from build123d import *

# Parameters (mm, degrees)
F0_R     = 3.663821
F0_R_2   = 3.4798
F1_DEPTH = 3.175


with BuildPart() as f1:
    # F0 (on Top) → F1 (new body)
    with BuildSketch(Plane.XY):
        with BuildLine():
            ThreePointArc((-89.269999, -19.05), (-87.410127, -23.540128), (-82.919999, -25.4))
            Line((-82.919999, -25.4), (56.780001, -25.4))
            ThreePointArc((56.780001, -25.4), (61.270129, -23.540128), (63.130001, -19.05))
            Line((63.130001, -19.05), (63.130001, -6.35))
            ThreePointArc((63.130001, -6.35), (61.270129, -1.859872), (56.780001, 0))
            Line((56.780001, 0), (-9.894999, 0))
            ThreePointArc((-9.894999, 0), (-14.385127, 1.859872), (-16.244999, 6.35))
            Line((-16.244999, 6.35), (-16.244999, 66.675))
            ThreePointArc((-16.244999, 66.675), (-18.104871, 71.165128), (-22.594999, 73.025))
            Line((-22.594999, 73.025), (-82.919999, 73.025))
            ThreePointArc((-82.919999, 73.025), (-87.410127, 71.165128), (-89.269999, 66.675))
            Line((-89.269999, 66.675), (-89.269999, -19.05))
        make_face()
        with BuildLine():
            Line((-66.204435, -12.7), (-78.904435, -12.7))
            ThreePointArc((-78.904435, -12.7), (-82.079435, -9.525), (-78.904435, -6.35))
            Line((-78.904435, -6.35), (-66.204435, -6.35))
            ThreePointArc((-66.204435, -6.35), (-63.029435, -9.525), (-66.204435, -12.7))
        make_face(mode=Mode.SUBTRACT)
        with BuildLine():
            Line((-14.559238, -12.7), (-27.259238, -12.7))
            ThreePointArc((-27.259238, -12.7), (-30.434238, -9.525), (-27.259238, -6.35))
            Line((-27.259238, -6.35), (-14.559238, -6.35))
            ThreePointArc((-14.559238, -6.35), (-11.384238, -9.525), (-14.559238, -12.7))
        make_face(mode=Mode.SUBTRACT)
        with Locations((44.080001, -9.525)):
            Circle(F0_R, mode=Mode.SUBTRACT)
        with Locations((-80.837199, 35.7378)):
            Circle(F0_R_2, mode=Mode.SUBTRACT)
        with Locations((-24.677799, 58.381684)):
            Circle(F0_R_2, mode=Mode.SUBTRACT)
    extrude(amount=F1_DEPTH)


solid = f1.part
Design review of the part built by this model. Coordinates are the model's own, in mm. A direction names the side the tool comes from. Coordinates: 2 decimals unless noted, no trailing zeros. Loops run counter-clockwise (first coordinate to the right, second up) from the corner with the lowest first, then second, coordinate; pieces in that order, holes last. Notation, with made-up numbers: M -19,2 L 27,2 A19 cw 27,30 Z; hole C 68.25,-28.75 d4. An arc over 180 degrees is marked long. Answer as CSV lines item,"result".
Item 1: Add section C-C on x = -2.5. State the section outline as (y, z) points (3 decimals).
Answer list:
outline,"M -25.4,0 L 0,0 L 0,3.175 L -25.4,3.175 Z"
Item 2: For P1, Ø1, axis at y = 26, z = 2.5, coming from the +X side (3 decimals); P2, Ø10, axis at x = 5.5, y = -9.5, coming from the -Z side; P3, Ø1, axis at x = 8, z = 2, coming from the +Y side, all flat-tipped, find the tip position at first contact; note any pin that passes through.
Answer list:
P1,"x = -16.245"
P2,"z = 0"
P3,"y = 0"
Item 3: Machinability: for faces 1 (the face through (-31, 14, 0)), 2 (the face through (-11.385, -9.455, 1.565)), 3 (the face through (-16.245, 36, 2)), which of the approach directions +Z, -Z, +X, -X, +Y, -Y give a long, thin tool a straight path to every point of the face, cutting with its end or side? Answer none if there is none.
Answer list:
face 1,"-Z, +X, -X, +Y, -Y"
face 2,"+Z, -Z"
face 3,"+Z, -Z, +X, +Y"
Item 4: Add section B-B on y = 50.5. State the section outline as (x, z) points (3 decimals), plus the area to 3 significant figures.
Answer list:
outline,"M -89.27,0 L -16.245,0 L -16.245,3.175 L -89.27,3.175 Z"
area,"232 mm²"
Item 5: For probe 1 along X at (y, z) = (-9.5, 1.95); probe 2 along Y at (x, z) = (-67.5, 1.45) (3 decimals); probe 3 along X at (y, z) = (58.5, 2.2) (3 decimals), list the stretches that pass through material, from the lowest coordinate up.
Answer list:
probe 1,"-89.27 to -82.08, -63.03 to -30.43, -11.38 to 40.42, 47.74 to 63.13"
probe 2,"-25.4 to -12.7, -6.35 to 73.025"
probe 3,"-89.27 to -28.156, -21.2 to -16.245"
Item 6: The part is to be moulded in two halves that separate along X. For faces 4 (the face through (-89.27, 24, 2)), 5 (the face through (-14, -25.4, 2)), 6 (the face through (-21, -6.35, 2)), 7 (the face through (-21, -12.7, 2)), say which applies: pulls with the +X half, pulls with the -X half, needs draft (parallel to the pull), parting line crosses it, or undercut.
Answer list:
face 4,"pulls with the -X half"
face 5,"needs draft"
face 6,"undercut"
face 7,"undercut"
Item 7: Add section A-A on z = 1.5. State the section outline as (x, y) points (3 decimals), plus the area to 3 significant figures.
Answer list:
outline,"M -89.27,-19.05 A6.35 ccw -82.92,-25.4 L 56.78,-25.4 A6.35 ccw 63.13,-19.05 L 63.13,-6.35 A6.35 ccw 56.78,0 L -9.895,0 A6.35 cw -16.245,6.35 L -16.245,66.675 A6.35 ccw -22.595,73.025 L -82.92,73.025 A6.35 ccw -89.27,66.675 Z; hole C -80.837,35.738 d6.96; hole M -78.904,-12.7 L -66.204,-12.7 A3.175 ccw -66.204,-6.35 L -78.904,-6.35 A3.175 ccw Z; hole C -24.678,58.382 d6.96; hole M -27.259,-12.7 L -14.559,-12.7 A3.175 ccw -14.559,-6.35 L -27.259,-6.35 A3.175 ccw Z; hole C 44.08,-9.525 d7.328"
area,"8,830 mm²"
